Source: CAD feature listing. Evaluate the final solid. Frame: model axes, mm. A direction names the side the tool comes from. Round coordinates to 2 decimals unless told otherwise and drop trailing zeros. Order: outer loops, then holes, each group sorted by start corner. A loop starts at its lowest first (then second) coordinate and runs counter-clockwise, first axis right, second up. Notation, with made-up numbers: (87, 13) -> (99, 13) arc R20 cw to (99, 52) -> close; hole circle Ø8 at (32, 43). An arc over 180 degrees is marked (long way). Write item = value, one per line. Start each with the question number.
(1) Contact query for flat-ended pins moving along their axis: pin 1 Ø2.5 at (x, y) = (10, 0) entering from -Z; pin 2 Ø6.5 at (x, y) = (1.5, 0.5) entering from +Z; pin 3 Ø1.5 at (y, z) = (5, -5) entering from -X. Output: stop coordinate, or through.
(2) Reachability of faces 4 (the face through (-12.5, 0, -6)), 5 (the face through (0, -3, -4)) from +Z, -Z, +X, -X, +Y, -Y: full face, straight path, thin tool, end or side. Return the list, or none.
(3) Cut plane A-A on x = 10.5. Return the cut outline in (y, z).
(4) Cut plane B-B on z = -7.5. Return the cut outline in (x, y), then the cut area to 3 significant figures.
(5) Draft query along X for faces 1 (the face through (-11.07, -5.5, -6.59)), 2 (the face through (-11.6, 0.07, -6.41)), 3 (the face through (11, 5.57, -6.59)). Return one class per face: released by +X, released by -X, zero draft, split by the parting line, or undercut.
(6) Ray query, line 1 (Y direction, x = 5, z = -6); line 2 (Z direction, x = -1.5, y = -1.75); line 3 (Y direction, x = 4, z = -9.25). Return the intervals inside material, ascending.
(7) Cut plane D-D on y = -4. Return the cut outline in (x, z).
(8) Cut plane C-C on x = -10. Return the cut outline in (y, z).
from build123d import *

# Parameters (mm, degrees)
F0_W     = 25
F0_H     = 14
F0_R     = 1.6
F0_W_2   = 11.5
F0_H_2   = 6
F0_R_2   = 1.25
F0_W_3   = 5
F0_H_3   = 2.5
F1_DEPTH = 13
F2_DEPTH = 9
F3_W     = 5
F3_H     = 2.5
F3_R     = 1.25
F4_DEPTH = 5
F4_TAPER = 9
F5_R     = 5


with BuildPart() as f1:
    # F0 (on Top) → F1 (new body)
    with BuildSketch(Plane.XY):
        Rectangle(F0_W, F0_H)
        with Locations((-10, 0)):
            Circle(F0_R, mode=Mode.SUBTRACT)
        with Locations((0.25, 0)):
            Rectangle(F0_W_2, F0_H_2, mode=Mode.SUBTRACT)
        with Locations((10, 0)):
            Circle(F0_R, mode=Mode.SUBTRACT)
        with Locations((0.25, 0)):
            Rectangle(F0_W_2, F0_H_2)
        with Locations((-2.5, 0)):
            Circle(F0_R_2, mode=Mode.SUBTRACT)
        with Locations((1.75, 0.0926498271)):
            Rectangle(F0_W_3, F0_H_3, mode=Mode.SUBTRACT)
        with Locations((-2.5, 0)):
            Circle(F0_R_2)
        with Locations((1.75, 0.0926498271)):
            Rectangle(F0_W_3, F0_H_3)
    extrude(amount=-F1_DEPTH)

    # F0 (on Top) → F2 (cut)
    with BuildSketch(Plane.XY):
        with Locations((0.25, 0)):
            Rectangle(F0_W_2, F0_H_2)
        with Locations((-2.5, 0)):
            Circle(F0_R_2, mode=Mode.SUBTRACT)
        with Locations((1.75, 0.0926498271)):
            Rectangle(F0_W_3, F0_H_3, mode=Mode.SUBTRACT)
        with Locations((-2.5, 0)):
            Circle(F0_R_2)
        with Locations((1.75, 0.0926498271)):
            Rectangle(F0_W_3, F0_H_3)
    extrude(amount=-F2_DEPTH, mode=Mode.SUBTRACT)

    # F3 (on face) → F4 (cut)
    with BuildSketch(Plane.XY.offset(-9)):
        with Locations((1.75, 0.0926498271)):
            Rectangle(F3_W, F3_H)
        with Locations((-2.5, 0)):
            Circle(F3_R)
    extrude(amount=-F4_DEPTH, taper=F4_TAPER, mode=Mode.SUBTRACT)

    # F5
    f5_edges = [f1.edges().sort_by_distance(p)[0] for p in [
        (-12.5, 7, -6.5),
        (12.5, -7, -6.5),
        (12.5, 7, -6.5),
        (-12.5, -7, -6.5),
    ]]
    fillet(f5_edges, radius=F5_R)


solid = f1.part
Evaluation:
q1.pin_1 = through
q1.pin_2 = 0
q1.pin_3 = -11.97
q2.face_4 = +Z, -Z, -X, +Y, -Y
q2.face_5 = +Z
q3.outline = (-6, -13) -> (-1.52, -13) -> (-1.52, 0) -> (-6, 0) -> close; (1.52, -13) -> (6, -13) -> (6, 0) -> (1.52, 0) -> close
q4.outline = (-12.5, -2) arc R5 ccw to (-7.5, -7) -> (7.5, -7) arc R5 ccw to (12.5, -2) -> (12.5, 2) arc R5 ccw to (7.5, 7) -> (-7.5, 7) arc R5 ccw to (-12.5, 2) -> close; hole circle Ø3.2 at (-10, 0); hole (-5.5, -3) -> (6, -3) -> (6, 3) -> (-5.5, 3) -> close; hole circle Ø3.2 at (10, 0)
q4.area = 243 mm^2
q5.face_1 = released by -X
q5.face_2 = undercut
q5.face_3 = released by +X
q6.line_1 = -7 to -3, 3 to 7
q6.line_2 = -13 to -9
q6.line_3 = -7 to -1.12, 1.3 to 7
q7.outline = (-12.08, -13) -> (12.08, -13) -> (12.08, 0) -> (-12.08, 0) -> close
q8.outline = (-6.33, -13) -> (-1.6, -13) -> (-1.6, 0) -> (-6.33, 0) -> close; (1.6, -13) -> (6.33, -13) -> (6.33, 0) -> (1.6, 0) -> close
